Here's the drawing with two shaded views (mm, measured from the low corner). I have some questions. A direction names the side the tool comes from. Coordinates: 2 decimals unless noted, no trailing zeros. Order: outer loops, then holes, each group sorted by start corner. A loop starts at its lowest first (then second) coordinate and runs counter-clockwise, first axis right, second up. Notation, with made-up numbers: (39, 50.25) -> (66, 50.25) arc R21 cw to (66, 87.25) -> close; hole circle Ø4 at (16, 84). An arc over 180 degrees is marked (long way). Answer as a JSON object with one key per item and string values. Group by question number.
(1) For pin 1 (2.5 mm diameter, centred on x = 17, y = 19.5, fed in from +Z); pin 2 (1 mm diameter, centred on x = 16.5, z = 5.5, fed in from +Y); pin 3 (3 mm diameter, centred on x = 3.5, z = 3.5, fed in from +Y); pin 4 (0.6 mm diameter, centred on x = 1.5, z = 4.5, fed in from -Y), each with a flat end and sliding along its axis, tell me the tip position at first contact or that it passes through.
(2) If we mould it in two halves opening along Y, with no side actions, what happens to the marked faces 4, 5, 6 and 7? For each: pulls with the +Y half, pulls with the -Y half, needs draft (parallel to the pull), parting line crosses it, or undercut.
(3) I want a section at B-B, the plane y = 5.5. List the corners of the cut face in (x, z) for me (1 decimal).
(4) I want a section at C-C, the plane z = 1.25. List the corners of the cut face in (x, y) for me.
(5) I want a section at D-D, the plane z = 3. List the corners of the cut face in (x, y) for me (1 decimal).
(6) Which directions (+Z, -Z, +X, -X, +Y, -Y) give clear straight access to the entire face, cutting with the end or side of a thin tool? Please do the marked faces 1, 2 and 3.
(7) I need wall thicknesses on line 1 (Y direction, x = 10.5, z = 6); line 2 (Y direction, x = 10.5, z = 3.25); line 3 (Y direction, x = 10.5, z = 2). Which ranges of each line are inside material? Lowest first, please.
(8) I want a section at A-A, the plane x = 10.5. List the corners of the cut face in (y, z) for me.
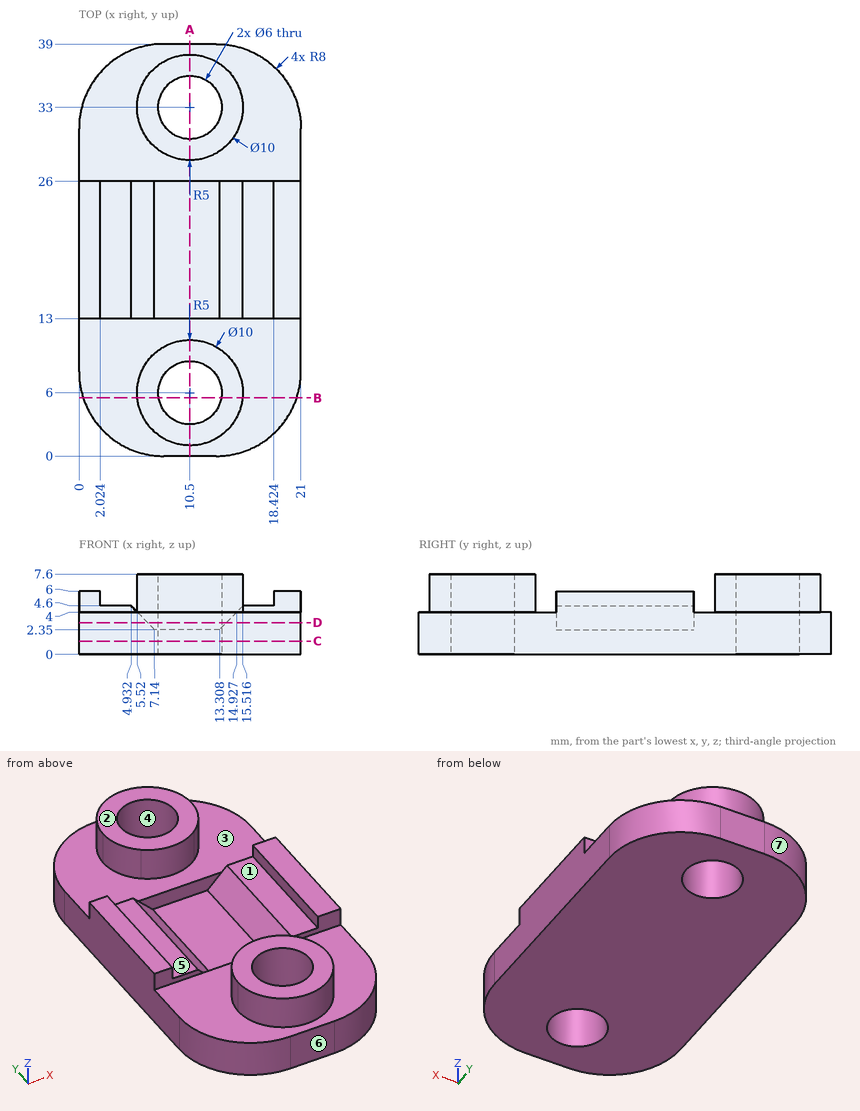
Computed values:
{
 "1": {"pin 1": "stops at z = 4.6", "pin 2": "passes through", "pin 3": "stops at y = 38.42", "pin 4": "stops at y = 13"},
 "2": {"face 4": "undercut", "face 5": "needs draft", "face 6": "pulls with the -Y half", "face 7": "pulls with the +Y half"},
 "3": {"outline": "(0.4, 0) -> (7.5, 0) -> (7.5, 7.6) -> (5.5, 7.6) -> (5.5, 4) -> (0.4, 4) -> close; (13.5, 0) -> (20.6, 0) -> (20.6, 4) -> (15.5, 4) -> (15.5, 7.6) -> (13.5, 7.6) -> close"},
 "4": {"outline": "(0, 8) arc R8 ccw to (8, 0) -> (13, 0) arc R8 ccw to (21, 8) -> (21, 31) arc R8 ccw to (13, 39) -> (8, 39) arc R8 ccw to (0, 31) -> close; hole circle Ø6 at (10.5, 6); hole circle Ø6 at (10.5, 33)"},
 "5": {"outline": "(0, 8) arc R8 ccw to (8, 0) -> (13, 0) arc R8 ccw to (21, 8) -> (21, 31) arc R8 ccw to (13, 39) -> (8, 39) arc R8 ccw to (0, 31) -> close; hole (6.5, 13) -> (13.9, 13) -> (13.9, 26) -> (6.5, 26) -> close; hole circle Ø6 at (10.5, 6); hole circle Ø6 at (10.5, 33)"},
 "6": {"face 1": "+Z, +Y, -Y", "face 2": "+Z, +X, -X, +Y, -Y", "face 3": "+Z"},
 "7": {"line 1": "y = 1 to 3, 9 to 11, 28 to 30, 36 to 38", "line 2": "y = 0 to 3, 9 to 13, 26 to 30, 36 to 39", "line 3": "y = 0 to 3, 9 to 30, 36 to 39"},
 "8": {"outline": "(0, 0) -> (3, 0) -> (3, 7.6) -> (1, 7.6) -> (1, 4) -> (0, 4) -> close; (9, 0) -> (30, 0) -> (30, 7.6) -> (28, 7.6) -> (28, 4) -> (26, 4) -> (26, 2.35) -> (13, 2.35) -> (13, 4) -> (11, 4) -> (11, 7.6) -> (9, 7.6) -> close; (36, 0) -> (39, 0) -> (39, 4) -> (38, 4) -> (38, 7.6) -> (36, 7.6) -> close"}
}
